from build123d import *

# Parameters (mm, degrees)
SKETCH1_W           = 80
SKETCH1_H           = 50
SKETCH1_R           = 2
BOSS_EXTRUDE1_DEPTH = 32
SKETCH2_R           = 6.5
CUT_EXTRUDE1_DEPTH  = 51


with BuildPart() as part:
    # Sketch1 → Boss-Extrude1 (new body)
    with BuildSketch(Plane(origin=(0, 0, 0), x_dir=(1, 0, 0), z_dir=(0, 1, 0))):
        with Locations((40, 25)):
            Rectangle(SKETCH1_W, SKETCH1_H)
        with Locations((10, 40)):
            Circle(SKETCH1_R, mode=Mode.SUBTRACT)
        with Locations((70, 40)):
            Circle(SKETCH1_R, mode=Mode.SUBTRACT)
        with Locations((70, 10)):
            Circle(SKETCH1_R, mode=Mode.SUBTRACT)
        with Locations((10, 10)):
            Circle(SKETCH1_R, mode=Mode.SUBTRACT)
    extrude(amount=BOSS_EXTRUDE1_DEPTH)

    # Sketch2 → Cut-Extrude1 (cut, through all)
    with BuildSketch(Plane.XY):
        with Locations((40, 16)):
            Circle(SKETCH2_R)
    extrude(amount=-CUT_EXTRUDE1_DEPTH, mode=Mode.SUBTRACT)


solid = part.part
The model under review builds one solid part; all positions refer to its coordinate system, in mm. Give positions to 0.01 mm unless a question says otherwise; leave off trailing zeros. Loops run counter-clockwise (first coordinate to the right, second up) from the corner with the lowest first, then second, coordinate; pieces in that order, holes last. Notation, with made-up numbers: (25.25, 85.5) -> (36.25, 85.5) arc R19 ccw to (36.25, 122.5) -> close; hole circle Ø7 at (0, -15.75). An arc over 180 degrees is marked (long way). Put each result on its own line as item: value. Start each with the question number.
1. Clearance check with a flat-ended pin moving along its axis: P1, Ø3.5, axis at x = 70, z = -40, coming from the +Y side. State where the tip first meets the part, or that it passes through.
2. Wall thickness on probe 1 along X at (y, z) = (25, -10); probe 2 along Z at (x, y) = (70, 7); probe 3 along X at (y, z) = (15.5, -21.5): over which ranges is each line inside the solid? List them lowest first.
3. We need section B-B on z = -40. State the section outline as (x, y) points, then the cut area to 3 significant figures.
4. We need section A-A on x = 70. State the section outline as (y, z) points, then the cut area to 3 significant figures.
5. We need section D-D on x = 40. State the section outline as (y, z) points.
6. Mouldability with a two-part tool opening along Y and no side actions: class faces 1 (the face through (33.506, 16.286, -24.65)), 2 (the face through (39, 0, -25)), 3 (the face through (0, 16, -25)), 4 (the face through (39, 32, -25)) as released by +Y, released by -Y, zero draft, split by the parting line, or undercut.
7. We need section C-C on y = 16. State the section outline as (x, z) points.
Determined:
1. P1: through
2. probe 1: 0 to 8, 12 to 68, 72 to 80
2. probe 2: -50 to -42, -38 to -12, -8 to 0
2. probe 3: 0 to 33.52, 46.48 to 80
3. outline: (0, 0) -> (8, 0) -> (8, 32) -> (0, 32) -> close; (12, 0) -> (68, 0) -> (68, 32) -> (12, 32) -> close; (72, 0) -> (80, 0) -> (80, 32) -> (72, 32) -> close; hole circle Ø13 at (40, 16)
3. area: 2,170 mm^2
4. outline: (0, -50) -> (32, -50) -> (32, -42) -> (0, -42) -> close; (0, -38) -> (32, -38) -> (32, -12) -> (0, -12) -> close; (0, -8) -> (32, -8) -> (32, 0) -> (0, 0) -> close
4. area: 1,340 mm^2
5. outline: (0, -50) -> (9.5, -50) -> (9.5, 0) -> (0, 0) -> close; (22.5, -50) -> (32, -50) -> (32, 0) -> (22.5, 0) -> close
6. face 1: undercut
6. face 2: released by -Y
6. face 3: zero draft
6. face 4: released by +Y
7. outline: (0, -50) -> (33.5, -50) -> (33.5, 0) -> (0, 0) -> close; (46.5, -50) -> (80, -50) -> (80, 0) -> (46.5, 0) -> close; hole circle Ø4 at (10, -40); hole circle Ø4 at (10, -10); hole circle Ø4 at (70, -40); hole circle Ø4 at (70, -10)
